Part print with two shaded views. Sizes in mm from the minimum x, y, z corner. A direction names the side the tool comes from. Coordinates: 2 decimals unless noted, no trailing zeros. Write each loop counter-clockwise with the first axis right and the second up, starting at its lowest first coordinate (ties: lowest second). Pieces come first, ordered by that corner, then holes. Notation, with made-up numbers: (24, 6.5) - (33, 6.5) arc R18 cw to (33, 26.5) - close; hole circle Ø9 at (-1.75, 88). An arc over 180 degrees is marked (long way). Answer in a Markdown table with one row per item. Add a question column.
Q1. Band-saw the part on D-D (y = 158). List the corners of the cut face in (x, z).
Q2. Drill centre lines: line 1 along Y through (x, z) = (11, 63); line 2 along Y through (x, z) = (9.75, 74.5). Where is each one in solid material? Low to high. Write a range as from..to.
Q3. 3-axis set-ups, long thin cutter, end or side, ignore diameter. For the marked faces 4 and 5: which of +Z, -Z, +X, -X, +Y, -Y reach the whole face in a straight line?
Q4. Pin check, flat tips, straight feed: pin 1 (2 mm diameter, centred on y = 48.5, z = 8, fed in from -X); pin 2 (6 mm diameter, centred on y = 155.5, z = 88, fed in from -X); pin 3 (2 mm diameter, centred on x = 4.5, z = 54.5, fed in from -Y). Stop position of each tip, or through.
Q5. Band-saw the part on A-A (z = 75). List the corners of the cut face in (x, y), and give its area (3 significant figures).
Q6. Band-saw the part on C-C (z = 12.5). List the corners of the cut face in (x, y).
Q7. Band-saw the part on B-B (x = 18). List the corners of the cut face in (y, z), and give its area (3 significant figures).
Q8. Two-plate mould, pull along Z, no slides. Class the marked faces 1, 2 and 3: +Z half, -Z half, draft (parallel to the pull), parting line (faces both ways), or undercut.
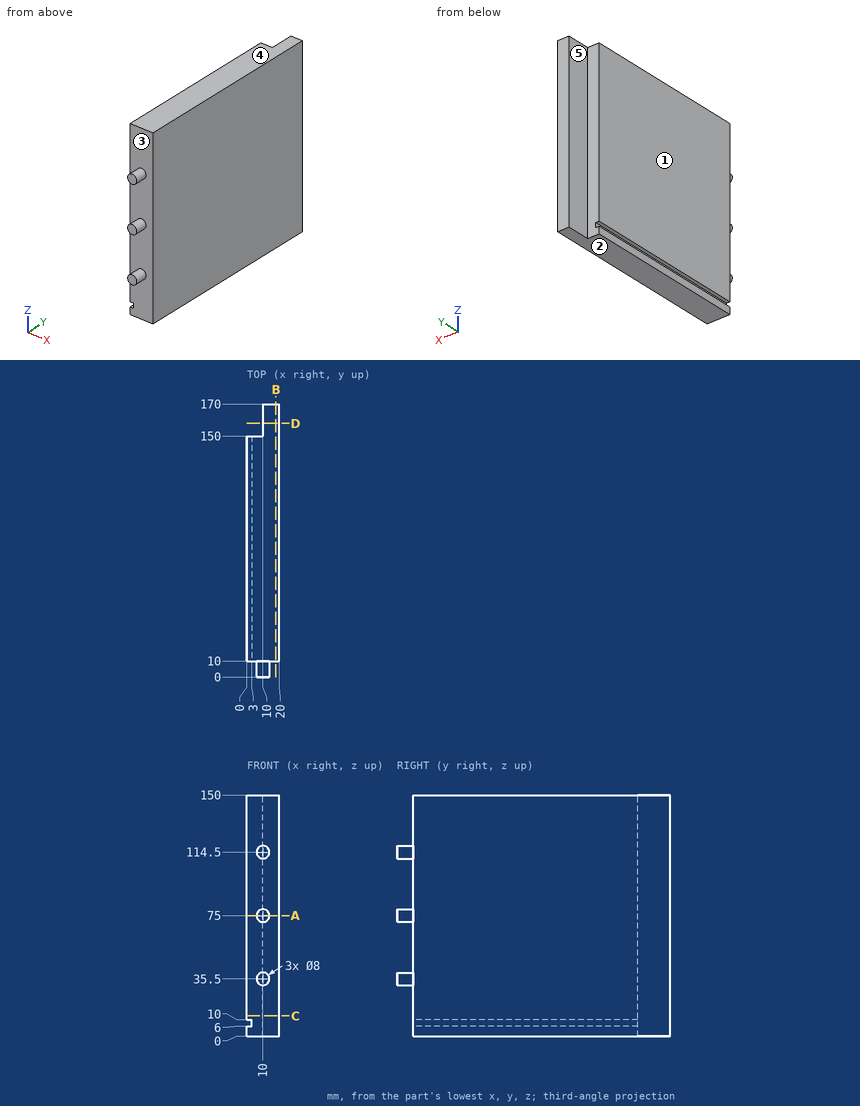
Checked values:
| question | item | result |
|---|---|---|
| 1 | outline | (10, 0) - (20, 0) - (20, 150) - (10, 150) - close |
| 2 | line 1 | y = 10..170 |
| 2 | line 2 | y = 0..150 |
| 3 | face 4 | +Z, +X, -X, +Y, -Y |
| 3 | face 5 | +Z, -Z, -X, +Y |
| 4 | pin 1 | stops at x = 3 |
| 4 | pin 2 | stops at x = 10 |
| 4 | pin 3 | stops at y = 10 |
| 5 | outline | (0, 10) - (6, 10) - (6, 0) - (14, 0) - (14, 10) - (20, 10) - (20, 170) - (10, 170) - (10, 150) - (0, 150) - close |
| 5 | area | 3,080 mm² |
| 6 | outline | (0, 10) - (20, 10) - (20, 170) - (10, 170) - (10, 150) - (0, 150) - close |
| 7 | outline | (10, 0) - (170, 0) - (170, 150) - (10, 150) - close |
| 7 | area | 24,000 mm² |
| 8 | face 1 | draft |
| 8 | face 2 | -Z half |
| 8 | face 3 | undercut |
